Part model, mm, in its own coordinate system. A direction names the side the tool comes from. Coordinates: 2 decimals unless noted, no trailing zeros. Order: outer loops, then holes, each group sorted by start corner. A loop starts at its lowest first (then second) coordinate and runs counter-clockwise, first axis right, second up.
```python
from build123d import *

# Parameters (mm, degrees)
SKETCH1_R                = 18
BOSS_EXTRUDE1_DEPTH      = 30
SKETCH2_R                = 12.5
BOSS_EXTRUDE2_DEPTH      = 30
BOSS_EXTRUDE2_DEPTH_BACK = 30
SKETCH3_R                = 11.5
CUT_EXTRUDE1_DEPTH       = 61.0000001


with BuildPart() as part:
    # Sketch1 → Boss-Extrude1 (new body)
    with BuildSketch(Plane(origin=(0, 0, 0), x_dir=(1, 0, 0), z_dir=(0, 1, 0))):
        Circle(SKETCH1_R)
    extrude(amount=BOSS_EXTRUDE1_DEPTH)

    # Sketch2 → Boss-Extrude2 (add, two sides)
    with BuildSketch(Plane.XY) as boss_extrude2_sk:
        with Locations((0, 15)):
            Circle(SKETCH2_R)
    extrude(amount=BOSS_EXTRUDE2_DEPTH)
    extrude(boss_extrude2_sk.sketch, amount=-BOSS_EXTRUDE2_DEPTH_BACK)

    # Sketch3 → Cut-Extrude1 (cut, through all)
    with BuildSketch(Plane.XY.offset(30)):
        with Locations((0, 15)):
            Circle(SKETCH3_R)
    extrude(amount=-CUT_EXTRUDE1_DEPTH, mode=Mode.SUBTRACT)


solid = part.part
```
(1) Slice it at B-B, the plane y = 15. Give the cut face in (x, z), then the cut area to 3 significant figures.
(2) Tool access for faces 1 (the face through (0, 0, 0)), 2 (the face through (-9.21, 23.45, -23.25)): list every direction of +Z, -Z, +X, -X, +Y, -Y with a clear straight run to the whole face (end or side of a thin tool).
(3) Pull direction Y, two halves, no side cores. Call faces 3 (the face through (4, 4, 30)), 4 (the face through (-9.21, 23.45, 23.25)), 5 (the face through (0, 30, 0)), 6 (the face through (-1.5, 26.4, 0.4)): +Y half, -Y half, draft (parallel to the pull), parting line (faces both ways), or undercut.
(4) Drop flat-ended pins along their axis: pin 1 (12 mm diameter, centred on x = -2, y = 15, fed in from +Z); pin 2 (8 mm diameter, centred on y = 6.5, z = -4.5, fed in from +X); pin 3 (8 mm diameter, centred on y = 13.5, z = -12, fed in from +X); pin 4 (3 mm diameter, centred on x = 12, z = 16.5, fed in from +Y). Give the stop position or say it passes through.
(5) Slice it at C-C, the plane z = 25. Give the cut face in (x, y), then the cut area to 3 significant figures.
(6) Slice it at D-D, the plane x = -8. Give the cut face in (y, z).
(7) Probe line 1 (Y direction, x = 0, z = 6); line 2 (Y direction, x = -9.5, z = 16); line 3 (X direction, y = 12, z = 5). List the from-to ranges inside material, lowest first.
(8) Slice it at A-A, the plane x = 0. Give the cut face in (y, z), then the cut area to 3 significant figures.
Here are the results:
1. outline: (-12.5, -30) - (-11.5, -30) - (-11.5, 30) - (-12.5, 30) - (-12.5, 12.95) arc R18 ccw to (-12.5, -12.95) - close; (11.5, -30) - (12.5, -30) - (12.5, -12.95) arc R18 ccw to (12.5, 12.95) - (12.5, 30) - (11.5, 30) - close
1. area: 317 mm2
2. face 1: +Z, -Z, +X, -X, -Y
2. face 2: -Z
3. face 3: draft
3. face 4: parting line
3. face 5: +Y half
3. face 6: undercut
4. pin 1: passes through
4. pin 2: stops at x = 17.99
4. pin 3: stops at x = 16.12
4. pin 4: stops at y = 21.78
5. outline: circle Ø25 at (0, 15); hole circle Ø23 at (0, 15)
5. area: 75.4 mm2
6. outline: (0, -16.12) - (5.4, -16.12) - (5.4, -30) - (6.74, -30) - (6.74, 30) - (5.4, 30) - (5.4, 16.12) - (0, 16.12) - close; (23.26, -30) - (24.6, -30) - (24.6, -16.12) - (30, -16.12) - (30, 16.12) - (24.6, 16.12) - (24.6, 30) - (23.26, 30) - close
7. line 1: y = 0 to 3.5, 26.5 to 30
7. line 2: y = 6.88 to 8.52, 21.48 to 23.12
7. line 3: x = -17.29 to -11.1, 11.1 to 17.29
8. outline: (0, -18) - (2.5, -18) - (2.5, -30) - (3.5, -30) - (3.5, 30) - (2.5, 30) - (2.5, 18) - (0, 18) - close; (26.5, -30) - (27.5, -30) - (27.5, -18) - (30, -18) - (30, 18) - (27.5, 18) - (27.5, 30) - (26.5, 30) - close
8. area: 300 mm2
